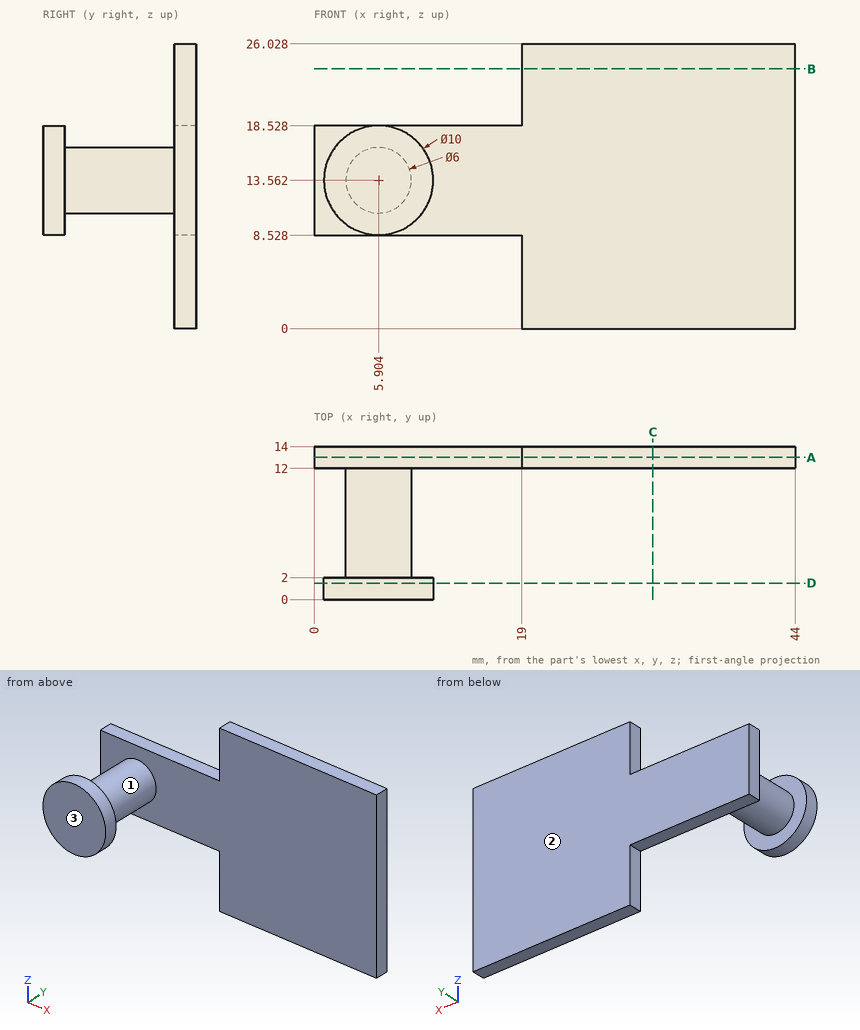
Print and shaded views of the part. All mm, measured from the part's lowest x, y and z. Coordinates: 2 decimals unless noted, no trailing zeros. Loops run counter-clockwise (first coordinate to the right, second up) from the corner with the lowest first, then second, coordinate; pieces in that order, holes last. Notation, with made-up numbers: M 67,-32.5 L 89,-32.5 A17 cw 89,-15.5 Z; hole C 40.25,78 d9. An arc over 180 degrees is marked long. Use a Markdown table: item, result. Add a question column.
Q1. Cut at D-D (y = 1.5). Write the cut outline in (x, z) (1 decimal).
Q2. Pin check, flat tips, straight feed: P1, Ø1.6, axis at x = 10, y = 13.5, coming from the +Z side; P2, Ø1, axis at y = 13, z = 2.5, coming from the -X side; P3, Ø3, axis at y = 5.5, z = 16, coming from the +X side. Stop position of each tip, or through.
Q3. Probe L1, parallel to Y at x = 9, z = 10; L2, parallel to X at y = 13.25, z = 20; L3, parallel to Y at x = 36.5, z = 23.75. List the from-to ranges inside material, lowest first.
Q4. Cut at C-C (x = 31). Write the cut outline in (y, z).
Q5. Cut at B-B (z = 23.75). Write the cut outline in (x, y), and give its area (3 significant figures).
Q6. Mould opens along Y. For the marked faces 1, 2 and 3 say: +Y half, -Y half, draft (parallel to the pull), parting line (faces both ways), or undercut.
Q7. Cut at A-A (y = 13). Write the cut outline in (x, z), and give its area (3 significant figures).
Worked out:
| question | item | result |
|---|---|---|
| 1 | outline | C 5.9,13.6 d10 |
| 2 | P1 | stops at z = 18.53 |
| 2 | P2 | stops at x = 19 |
| 2 | P3 | stops at x = 8.75 |
| 3 | L1 | y = 0 to 2, 12 to 14 |
| 3 | L2 | x = 19 to 44 |
| 3 | L3 | y = 12 to 14 |
| 4 | outline | M 12,0 L 14,0 L 14,26.03 L 12,26.03 Z |
| 5 | outline | M 19,12 L 44,12 L 44,14 L 19,14 Z |
| 5 | area | 50.0 mm2 |
| 6 | face 1 | undercut |
| 6 | face 2 | +Y half |
| 6 | face 3 | -Y half |
| 7 | outline | M 0,8.53 L 19,8.53 L 19,0 L 44,0 L 44,26.03 L 19,26.03 L 19,18.53 L 0,18.53 Z |
| 7 | area | 841 mm2 |
